Read the model definition and answer for the solid it produces. Units are mm, in the model's axes. Face numbers are marked on the shaded views. A direction names the side the tool comes from. Coordinates: 2 decimals unless noted, no trailing zeros. Write each loop counter-clockwise with the first axis right and the second up, starting at its lowest first coordinate (ties: lowest second). Pieces come first, ordered by that corner, then holes. Notation, with made-up numbers: (82, 80) -> (118, 80) arc R15 ccw to (118, 107) -> close; hole circle Ø10 at (83.25, 58). An arc over 180 degrees is marked (long way). One line per item, written item: value. Start each with the question number.
1. Given P1, Ø5, axis at x = -36, z = -23, coming from the -Y side; P2, Ø3, axis at x = -25, y = 6, coming from the +Z side; P3, Ø2, axis at x = -43, y = 6, coming from the -Z side; P4, Ø2, axis at y = 9, z = -29.5, coming from the -X side, each flat-ended and moving along its own axis, determine where each tip first touches the part or whether it passes through.
2. Find section C-C, the plane x = -44.5. Write down the section's boundary in (y, z).
3. For the marked faces 1 and 2, determine the directions among +Z, -Z, +X, -X, +Y, -Y from which every point of the face is accessible in a straight line to the end or side of a thin tool.
4. Find section D-D, the plane z = -51. Write down the section's boundary in (x, y).
5. Consider line 1 along Z through (x, y) = (-57, 0.3); line 2 along X through (y, z) = (0.7, -3); line 3 along Z through (x, y) = (-17, 10.5). Determine where each line is inside the solid, lowest interval first.
6. Find section B-B, the plane z = -97. Write down the section's boundary in (x, y).
7. Find section A-A, the plane x = -3. Write down the section's boundary in (y, z).
Autodesk Inventor part; units mm, degrees
ref_plane "Work Plane1" through (-50, 1.6, -50) normal (0, 0, 1) x (1, 0, 0)
ref_plane "YZ Plane" through (0, 0, 0) normal (1, 0, 0) x (0, 1, 0)
ref_plane "XZ Plane" through (0, 0, 0) normal (0, 1, 0) x (-1, 0, 0)
sketch "Sketch1" plane through (0, 0, 0) normal (0, 1, 0) x (-1, 0, 0)
  line L0 (0, 0) -> (60, 0)
  line L1 (60, 0) -> (60, -100)
  line L2 (60, -100) -> (0, -100)
  line L3 (0, -100) -> (0, 0)
  dimension "d0" = 60
  dimension "d1" = 100
extrude "Extrusion1" add sketch "Sketch1" along normal blind 1.6
sketch "Sketch2" plane through (0, 1.6, 0) normal (0, 1, 0) x (1, 0, 0)
  line L0 (-60, 0) -> (0, 0)
  line L1 (0, 0) -> (0, 100)
  point P0 (-3, 3)
  point P1 (-57, 3)
  point P2 (-3, 97)
  point P3 (-57, 97)
  dimension "d4" = 3
  dimension "d5" = 3
  dimension "d8" = 54
  dimension "d11" = 94
hole "Hole1" at (-3, 1.6, -3) at (-57, 1.6, -3) at (-3, 1.6, -97) at (-57, 1.6, -97) direction (0, -1, 0) diameter 3.4 end through all
sketch "Sketch3" plane through (0, 1.6, 0) normal (0, 1, 0) x (1, 0, 0)
  line L0 (0, 0) -> (-60, 0) construction
  line L1 (-30, 0) -> (-30, 100) construction
  line L2 (-60, 100) -> (0, 100) construction
  line L3 (-50, 1) -> (-10, 1)
  line L4 (-10, 1) -> (-10, 99)
  line L5 (-10, 99) -> (-50, 99)
  line L6 (-50, 99) -> (-50, 1)
  line L7 (-50, 1) -> (-10, 99) construction
  point P0 (-30, 50)
  dimension "d21" = 40
  dimension "d22" = 98
extrude "Extrusion2" add sketch "Sketch3" along normal blind 10
ref_plane "Work Plane1" through (-50, 1.6, -50) normal (0, 0, 1) x (1, 0, 0)
properties part number "LCD Screen"
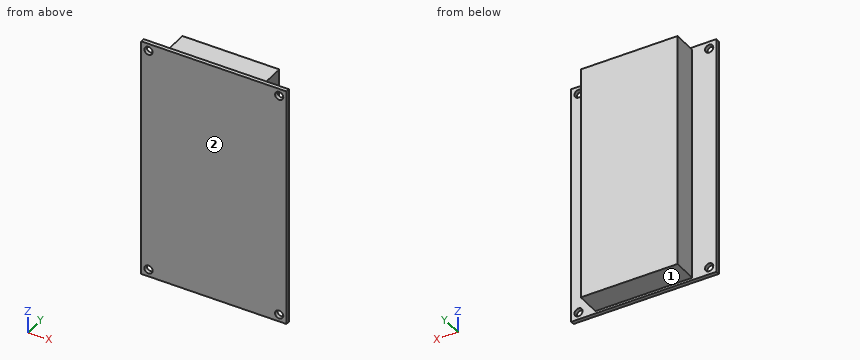
Answer block:
1. P1: stops at y = 0
1. P2: stops at z = -1
1. P3: stops at z = -99
1. P4: stops at x = -50
2. outline: (0, -100) -> (1.6, -100) -> (1.6, -99) -> (11.6, -99) -> (11.6, -1) -> (1.6, -1) -> (1.6, 0) -> (0, 0) -> close
3. face 1: -Z, +X, -X, +Y
3. face 2: +Z, -Z, +X, -X, -Y
4. outline: (-60, 0) -> (0, 0) -> (0, 1.6) -> (-10, 1.6) -> (-10, 11.6) -> (-50, 11.6) -> (-50, 1.6) -> (-60, 1.6) -> close
5. line 1: z = -100 to -98.7, -95.3 to -4.7, -1.3 to 0
5. line 2: x = -60 to -58.7, -55.3 to -4.7, -1.3 to 0
5. line 3: z = -99 to -1
6. outline: (-60, 0) -> (-58.7, 0) -> (-58.7, 1.6) -> (-60, 1.6) -> close; (-55.3, 0) -> (-4.7, 0) -> (-4.7, 1.6) -> (-10, 1.6) -> (-10, 11.6) -> (-50, 11.6) -> (-50, 1.6) -> (-55.3, 1.6) -> close; (-1.3, 0) -> (0, 0) -> (0, 1.6) -> (-1.3, 1.6) -> close
7. outline: (0, -100) -> (1.6, -100) -> (1.6, -98.7) -> (0, -98.7) -> close; (0, -95.3) -> (1.6, -95.3) -> (1.6, -4.7) -> (0, -4.7) -> close; (0, -1.3) -> (1.6, -1.3) -> (1.6, 0) -> (0, 0) -> close
